Geometry check sheet. Reference: the model listing, model coordinates, mm. Give positions to 0.01 mm unless a question says otherwise; leave off trailing zeros. Order: outer loops, then holes, each group sorted by start corner. A loop starts at its lowest first (then second) coordinate and runs counter-clockwise, first axis right, second up. Notation, with made-up numbers: M 15,0.25 L 45,0.25 A14 cw 45,23.25 Z; hole C 30.5,52.25 d6. An arc over 180 degrees is marked long. Put each result on its own line as item: value. Start each with the question number.
Q1. Go/stop test with flat-tipped pins: pin 1 (5 mm diameter, centred on x = 36.92, y = 20.73, fed in from -Z); pin 2 (2 mm diameter, centred on y = -17, z = 3, fed in from -X) (3 decimals). Record where each tip stops, or that it passes through.
Q2. Section check C-C on z = 2.65. Record the cut outline in (x, y), then the cut area to 3 significant figures.
Q3. Section check A-A on x = 34.5. Record the cut outline in (y, z), then the cut area to 3 significant figures.
Q4. Material ranges on L1, parallel to X at y = 0, z = 2.35; L2, parallel to Y at x = 0, z = 3.05; L3, parallel to X at y = -2.5, z = 0.6, recorded low to high.
Q5. Section check B-B on y = -4.5. Record the cut outline in (x, z), then the cut area to 3 significant figures.
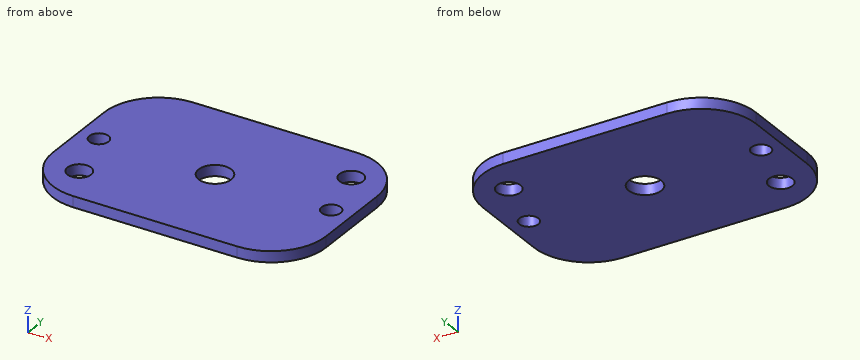
```python
from build123d import *

# Parameters (mm, degrees)
F0_W      = 100
F0_H      = 70
F3_DEPTH  = 4
F2_R      = 4.322492
F4_DEPTH  = 5
F1_R      = 3.5
F5_DEPTH  = 5
F6_R      = 20
F7_R      = 20
F8_R      = 20
F9_R      = 20
F10_R     = 6
F11_DEPTH = 5


with BuildPart() as f3:
    # F0 (on Top) → F3 (new body)
    with BuildSketch(Plane.XY):
        Rectangle(F0_W, F0_H)
    extrude(amount=F3_DEPTH)

    # F2 (on Top) → F4 (cut)
    with BuildSketch(Plane.XY):
        with Locations((36.918391, 20.728212)):
            Circle(F2_R)
        with Locations((-36.812667, -20.548884)):
            Circle(F2_R)
    extrude(amount=F4_DEPTH, mode=Mode.SUBTRACT)

    # F1 (on face) → F5 (cut)
    with BuildSketch(Plane.XY):
        with Locations((-42.48777, 0)):
            Circle(F1_R)
        with Locations((42.51223, 0)):
            Circle(F1_R)
    extrude(amount=F5_DEPTH, mode=Mode.SUBTRACT)

    # F6
    f6_edges = [f3.edges().sort_by_distance(p)[0] for p in [
        (-50, -35, 2),
    ]]
    fillet(f6_edges, radius=F6_R)

    # F7
    f7_edges = [f3.edges().sort_by_distance(p)[0] for p in [
        (50, 35, 2),
    ]]
    fillet(f7_edges, radius=F7_R)

    # F8
    f8_edges = [f3.edges().sort_by_distance(p)[0] for p in [
        (50, -35, 2),
    ]]
    fillet(f8_edges, radius=F8_R)

    # F9
    f9_edges = [f3.edges().sort_by_distance(p)[0] for p in [
        (-50, 35, 2),
    ]]
    fillet(f9_edges, radius=F9_R)

    # F10 (on face) → F11 (cut)
    with BuildSketch(Plane(origin=(0, 0, 0), x_dir=(1, 0, 0), z_dir=(0, 0, -1))):
        Circle(F10_R)
    extrude(amount=-F11_DEPTH, mode=Mode.SUBTRACT)


solid = f3.part
```
Results found:
1. pin 1: passes through
1. pin 2: stops at x = -49.975
2. outline: M -50,-15 A20 ccw -30,-35 L 30,-35 A20 ccw 50,-15 L 50,15 A20 ccw 30,35 L -30,35 A20 ccw -50,15 Z; hole C -42.49,0 d7; hole C -36.81,-20.55 d8.64; hole C 0,0 d12; hole C 36.92,20.73 d8.64; hole C 42.51,0 d7
2. area: 6,350 mm^2
3. outline: M -34.49,0 L 17.15,0 L 17.15,4 L -34.49,4 Z; M 24.31,0 L 34.49,0 L 34.49,4 L 24.31,4 Z
3. area: 247 mm^2
4. L1: x = -50 to -45.99, -38.99 to -6, 6 to 39.01, 46.01 to 50
4. L2: y = -35 to -6, 6 to 35
4. L3: x = -50 to -44.94, -40.04 to -5.45, 5.45 to 40.06, 44.96 to 50
5. outline: M -50,0 L -3.97,0 L -3.97,4 L -50,4 Z; M 3.97,0 L 50,0 L 50,4 L 3.97,4 Z
5. area: 368 mm^2
